CAD build for the part. Positions are in the model's coordinates, mm. Give positions to 0.01 mm unless a question says otherwise; leave off trailing zeros. Order: outer loops, then holes, each group sorted by start corner. A loop starts at its lowest first (then second) coordinate and runs counter-clockwise, first axis right, second up.
Item 1: Wall check: L1, parallel to Z at x = -458, y = -6; L2, parallel to Z at x = -221, y = -10.75; L3, parallel to Y at x = -115, z = 68. Give the ranges that are in metal, low to high.
Item 2: Flat gauge pins, fed straight in: P1, Ø4, axis at x = 301.5, y = -11.5, coming from the +Z side; P2, Ø4, axis at x = -324, y = -3.5, coming from the -Z side; P3, Ø3, axis at x = -364, z = 72, coming from the -Y side. Where does each tip first touch, or does it go through?
Item 3: Band-saw the part on B-B on y = -4. Give the cut face in (x, z).
Item 4: Band-saw the part on A-A on x = 541. Give the cut face in (y, z) (3 decimals).
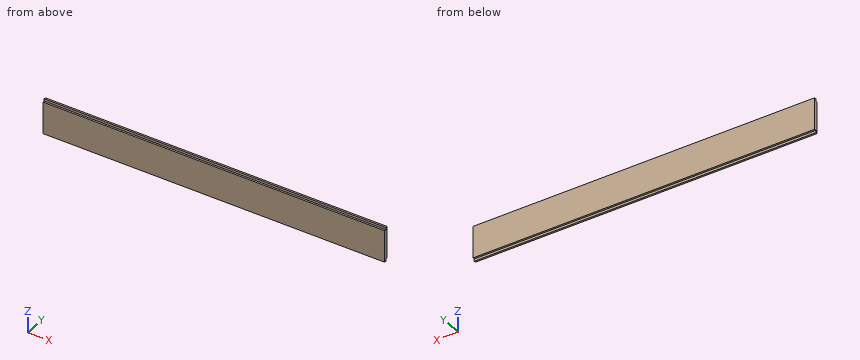
```python
from build123d import *

# Parameters (mm, degrees)
F1_DEPTH = 15.875
F2_W     = 8.001
F2_H     = 10.414
F3_DEPTH = 1524


with BuildPart() as f1:
    # F0 (on Front) → F1 (new body)
    with BuildSketch(Plane.XZ):
        Polygon((762, -76.2), (762, 0), (762, 76.2), (-762, 76.2), (-762, -76.2), align=None)
    extrude(amount=F1_DEPTH)

    # F2 (on face) → F3 (cut, through all)
    with BuildSketch(Plane.YZ.offset(762)):
        with Locations((-4.0005, -70.993)):
            Rectangle(F2_W, F2_H)
        with Locations((-11.8745, 70.993)):
            Rectangle(F2_W, F2_H)
    extrude(amount=-F3_DEPTH, mode=Mode.SUBTRACT)


solid = f1.part
```
The answers:
1. L1: z = -65.79 to 76.2
1. L2: z = -76.2 to 65.79
1. L3: y = -7.87 to 0
2. P1: stops at z = 65.79
2. P2: stops at z = -65.79
2. P3: stops at y = -7.87
3. outline: (-762, -65.79) - (762, -65.79) - (762, 76.2) - (-762, 76.2) - close
4. outline: (-15.875, -76.2) - (-8.001, -76.2) - (-8.001, -65.786) - (0, -65.786) - (0, 76.2) - (-7.874, 76.2) - (-7.874, 65.786) - (-15.875, 65.786) - close
